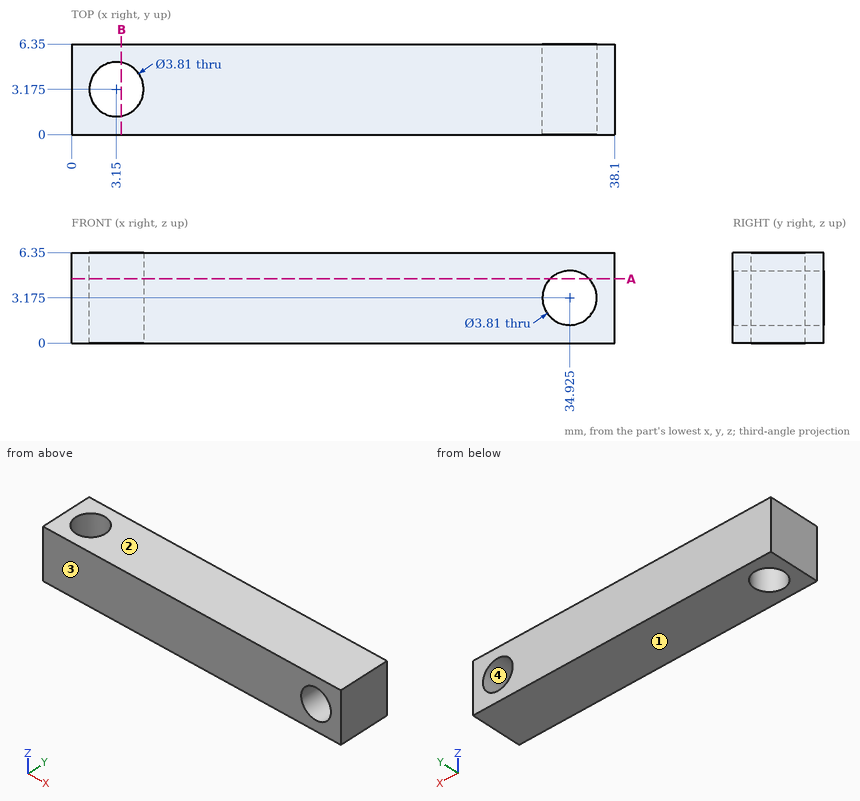
Verification items for this drawing (mm, ordinates from the low corner). Give positions to 0.01 mm unless a question says otherwise; leave off trailing zeros. Loops run counter-clockwise (first coordinate to the right, second up) from the corner with the lowest first, then second, coordinate; pieces in that order, holes last.
1. Go/stop test with a flat-tipped pin: P1, Ø2.5, axis at x = 34.925, z = 3.175, coming from the -Y side. Record where the tip stops, or that it passes through.
Derived:
P1: passes through
2. Material ranges on probe 1 along X at (y, z) = (4, 2) (1 decimal); probe 2 along X at (y, z) = (3, 1); probe 3 along X at (y, z) = (5.5, 4.5) (1 decimal), recorded low to high.
Derived:
probe 1: x = 0 to 1.4, 4.9 to 33.4, 36.4 to 38.1
probe 2: x = 0 to 1.25, 5.05 to 38.1
probe 3: x = 0 to 33.6, 36.3 to 38.1
3. Cross-section at B-B on x = 3.5. Record the cut outline in (y, z).
Derived:
outline: (0, 0) - (1.3, 0) - (1.3, 6.35) - (0, 6.35) - close; (5.05, 0) - (6.35, 0) - (6.35, 6.35) - (5.05, 6.35) - close
4. Release check for a two-part mould opening along Z. For the marked faces 1, 2, 3 and 4 record: +Z half, -Z half, draft (parallel to the pull), parting line (faces both ways), or undercut.
Derived:
face 1: -Z half
face 2: +Z half
face 3: draft
face 4: undercut
5. Cross-section at A-A on z = 4.5. Count the separate pieces of the cut face and the enclosed holes in it, and give its area (3 significant figures).
Derived:
separate pieces: 2
enclosed holes: 1
area: 213 mm2
